Here's how the part is built. I have some questions about the finished solid (model axes, mm). A direction names the side the tool comes from. Round coordinates to 2 decimals unless told otherwise and drop trailing zeros. Write each loop counter-clockwise with the first axis right and the second up, starting at its lowest first coordinate (ties: lowest second). Pieces come first, ordered by that corner, then holes. Notation, with made-up numbers: (45.5, 81.5) - (81.5, 81.5) arc R17 ccw to (81.5, 107.5) - close; hole circle Ø2 at (48.25, 70). An arc over 180 degrees is marked (long way). Use one line per item in the form item = value. Start each with the question number.
1. I want a section at C-C, the plane x = -13.5. List the corners of the cut face in (y, z) for me, plus the area to 3 significant figures.
2. I want a section at B-B, the plane y = 2.5. List the corners of the cut face in (x, z) for me.
3. I want a section at A-A, the plane z = -3.75. State how many separate pieces and enclosed holes the cut face has, plus the area to 3 significant figures.
4. If I drill on line 1 along X through (y, z) = (-13, -0.5); line 2 along Y through (x, z) = (115, 5); line 3 along X through (y, z) = (73, -1.5), over which ranges is the centre line in solid material (lowest first)?
5. Will these pins go through, and if not, where does the flat tip stop? pin 1 (1.2 mm diameter, centred on x = -114, y = 80, fed in from +Z); pin 2 (8 mm diameter, centred on x = 87, z = -3.5, fed in from -Y); pin 3 (11 mm diameter, centred on x = -85.5, z = -4, fed in from -Y).
6. Which directions (+Z, -Z, +X, -X, +Y, -Y) give clear straight access to the entire face, cutting with the end or side of a thin tool? Please do faces 1 (the flat face through (35, 101.846, -5)), 2 (the flat face through (100, -23, -5)), 3 (the flat face through (70, -1, -5)), 4 (the flat face through (35, -106.335, -5)), 5 (the cylindrical face through (-94.677, 80.816, -4.93)).
```python
from build123d import *

# Parameters (mm, degrees)
EXTRUDE_1_DEPTH     = 10
SKETCH_2_R          = 2
CUT_EXTRUDE_1_DEPTH = 8
EXTRUDE_2_DEPTH     = 10


with BuildPart() as part:
    # 草图1 → 凸台-拉伸1 (new body)
    with BuildSketch(Plane.XY):
        with BuildLine():
            Line((-75, -125), (75, -125))
            ThreePointArc((75, -125), (110.355339059, -110.355339059), (125, -75))
            Line((125, -75), (125, 75))
            ThreePointArc((125, 75), (110.355339059, 110.355339059), (75, 125))
            Line((75, 125), (-75, 125))
            ThreePointArc((-75, 125), (-110.355339059, 110.355339059), (-125, 75))
            Line((-125, 75), (-125, -75))
            ThreePointArc((-125, -75), (-110.355339059, -110.355339059), (-75, -125))
        make_face()
    extrude(amount=EXTRUDE_1_DEPTH)

    # 草图2 → 切除-拉伸1 (cut)
    with BuildSketch(Plane.XY.offset(10)):
        with Locations((115, 80)):
            Circle(SKETCH_2_R)
        with Locations((85, 80)):
            Circle(SKETCH_2_R)
        with Locations((115, -80)):
            Circle(SKETCH_2_R)
        with Locations((85, -80)):
            Circle(SKETCH_2_R)
        with Locations((-115, -80)):
            Circle(SKETCH_2_R)
        with Locations((-85, -80)):
            Circle(SKETCH_2_R)
        with Locations((-85, 80)):
            Circle(SKETCH_2_R)
        with Locations((-115, 80)):
            Circle(SKETCH_2_R)
    extrude(amount=-CUT_EXTRUDE_1_DEPTH, mode=Mode.SUBTRACT)

    # 草图3 → 凸台-拉伸2 (add)
    with BuildSketch(Plane(origin=(0, 0, 0), x_dir=(-1, 0, 0), z_dir=(0, 0, -1))):
        with BuildLine():
            Line((-20, 96.846443928), (-20, -101.335336728))
            ThreePointArc((-20, -101.335336728), (-21.464466094, -104.870870634), (-25, -106.335336728))
            Line((-25, -106.335336728), (-45, -106.335336728))
            ThreePointArc((-45, -106.335336728), (-48.535533906, -104.870870634), (-50, -101.335336728))
            Line((-50, -101.335336728), (-50, 96.846443928))
            ThreePointArc((-50, 96.846443928), (-48.535533906, 100.381977834), (-45, 101.846443928))
            Line((-45, 101.846443928), (-25, 101.846443928))
            ThreePointArc((-25, 101.846443928), (-21.464466094, 100.381977834), (-20, 96.846443928))
        make_face()
        with BuildLine():
            Line((-70, 96.846443928), (-70, -101.335336728))
            ThreePointArc((-70, -101.335336728), (-71.464466094, -104.870870634), (-75, -106.335336728))
            Line((-75, -106.335336728), (-95, -106.335336728))
            ThreePointArc((-95, -106.335336728), (-98.535533906, -104.870870634), (-100, -101.335336728))
            Line((-100, -101.335336728), (-100, 57.613560287))
            ThreePointArc((-100, 57.613560287), (-94.783283784, 80.504296116), (-85, 101.846443928))
            Line((-85, 101.846443928), (-75, 101.846443928))
            ThreePointArc((-75, 101.846443928), (-71.464466094, 100.381977834), (-70, 96.846443928))
        make_face()
        with BuildLine():
            Line((45, -106.335336728), (25, -106.335336728))
            ThreePointArc((25, -106.335336728), (21.464466094, -104.870870634), (20, -101.335336728))
            Line((20, -101.335336728), (20, 96.846443928))
            ThreePointArc((20, 96.846443928), (21.464466094, 100.381977834), (25, 101.846443928))
            Line((25, 101.846443928), (45, 101.846443928))
            ThreePointArc((45, 101.846443928), (48.535533906, 100.381977834), (50, 96.846443928))
            Line((50, 96.846443928), (50, -101.335336728))
            ThreePointArc((50, -101.335336728), (48.535533906, -104.870870634), (45, -106.335336728))
        make_face()
        with BuildLine():
            Line((95, -106.335336728), (75, -106.335336728))
            ThreePointArc((75, -106.335336728), (71.464466094, -104.870870634), (70, -101.335336728))
            Line((70, -101.335336728), (70, 96.846443928))
            ThreePointArc((70, 96.846443928), (71.464466094, 100.381977834), (75, 101.846443928))
            Line((75, 101.846443928), (85, 101.846443928))
            ThreePointArc((85, 101.846443928), (94.783283784, 80.504296116), (100, 57.613560287))
            Line((100, 57.613560287), (100, -101.335336728))
            ThreePointArc((100, -101.335336728), (98.535533906, -104.870870634), (95, -106.335336728))
        make_face()
    extrude(amount=EXTRUDE_2_DEPTH)


solid = part.part
```
Model answer:
q1.outline = (-125, 0) - (125, 0) - (125, 10) - (-125, 10) - close
q1.area = 2,500 mm2
q2.outline = (-125, 0) - (-100, 0) - (-100, -10) - (-70, -10) - (-70, 0) - (-50, 0) - (-50, -10) - (-20, -10) - (-20, 0) - (20, 0) - (20, -10) - (50, -10) - (50, 0) - (70, 0) - (70, -10) - (100, -10) - (100, 0) - (125, 0) - (125, 10) - (-125, 10) - close
q3.separate_pieces = 4
q3.enclosed_holes = 0
q3.area = 24,400 mm2
q4.line_1 = -100 to -70, -50 to -20, 20 to 50, 70 to 100
q4.line_2 = -105 to -82, -78 to 78, 82 to 105
q4.line_3 = -97.04 to -70, -50 to -20, 20 to 50, 70 to 97.04
q5.pin_1 = 2
q5.pin_2 = -123.98
q5.pin_3 = -124.55
q6.face_1 = -Z, +X, -X, +Y
q6.face_2 = -Z, +X, +Y, -Y
q6.face_3 = -Z, +Y, -Y
q6.face_4 = -Z, +X, -X, -Y
q6.face_5 = -Z, -X, +Y
